```python
from build123d import *

# Parameters (mm, degrees)
F1_DEPTH  = 22
F0_R      = 28.575
F2_DEPTH  = 32
F3_W      = 22
F3_H      = 50
F4_DEPTH  = 114
F5_R      = 11.1
F6_DEPTH  = 32.001
F8_DEPTH  = 10
F9_DEPTH  = 64.001
F10_SIZE2 = 12
F10_SIZE  = 12


with BuildPart() as f1:
    # F0 (on Front) → F1 (new body, symmetric)
    with BuildSketch(Plane.XZ):
        with BuildLine():
            ThreePointArc((35.142567, 41), (49.05965, 22.564368), (54, 0))
            ThreePointArc((54, 0), (49.05965, -22.564368), (35.142567, -41))
            Line((35.142567, -41), (174, -41))
            Line((174, -41), (174, 41))
            Line((174, 41), (35.142567, 41))
        make_face()
    extrude(amount=F1_DEPTH, both=True)

    # F0 (on Front) → F2 (join, symmetric)
    with BuildSketch(Plane.XZ):
        with BuildLine():
            ThreePointArc((35.142567, -41), (49.05965, -22.564368), (54, 0))
            ThreePointArc((54, 0), (49.05965, 22.564368), (35.142567, 41))
            ThreePointArc((35.142567, 41), (-54, 0), (35.142567, -41))
        make_face()
        Circle(F0_R, mode=Mode.SUBTRACT)
        Circle(F0_R)
    extrude(amount=F2_DEPTH, both=True)

    # F3 (on face) → F4 (cut)
    with BuildSketch(Plane.YZ.offset(174)):
        with Locations((-11, 0)):
            Rectangle(F3_W, F3_H)
    extrude(amount=-F4_DEPTH, mode=Mode.SUBTRACT)

    # F5 (on face) → F6 (cut, through all)
    with BuildSketch(Plane.XZ):
        with Locations((139, 0)):
            Circle(F5_R)
        with Locations((89, 0)):
            Circle(F5_R)
    extrude(amount=-F6_DEPTH, mode=Mode.SUBTRACT)

    # F7 (on face) → F8 (join)
    with BuildSketch(Plane.XZ.offset(32)):
        with BuildLine():
            ThreePointArc((-23.675528, -16), (-28.575, 0), (-23.675528, 16))
            Line((-23.675528, 16), (-51.575188, 16))
            ThreePointArc((-51.575188, 16), (-54, 0), (-51.575188, -16))
            Line((-51.575188, -16), (-23.675528, -16))
        make_face()
        with BuildLine():
            ThreePointArc((23.675528, 16), (27.322691, 8.366672), (28.575, 0))
            ThreePointArc((28.575, 0), (27.322691, -8.366672), (23.675528, -16))
            Line((23.675528, -16), (51.575188, -16))
            ThreePointArc((51.575188, -16), (53.390356, -8.091349), (54, 0))
            ThreePointArc((54, 0), (53.390356, 8.091349), (51.575188, 16))
            Line((51.575188, 16), (23.675528, 16))
        make_face()
    extrude(amount=F8_DEPTH)

    # F7 (on face) → F9 (cut, through all)
    with BuildSketch(Plane.XZ.offset(32)):
        with BuildLine():
            ThreePointArc((23.675528, -16), (27.322691, -8.366672), (28.575, 0))
            ThreePointArc((28.575, 0), (27.322691, 8.366672), (23.675528, 16))
            ThreePointArc((23.675528, 16), (0, 28.575), (-23.675528, 16))
            ThreePointArc((-23.675528, 16), (-28.575, 0), (-23.675528, -16))
            ThreePointArc((-23.675528, -16), (0, -28.575), (23.675528, -16))
        make_face()
    extrude(amount=-F9_DEPTH, mode=Mode.SUBTRACT)

    # F10
    f10_edges = [f1.edges().sort_by_distance(p)[0] for p in [
        (174, -22, -33),
        (174, -22, 33),
    ]]
    chamfer(f10_edges, length=F10_SIZE, length2=F10_SIZE2)


solid = f1.part
```
Read the model definition and answer for the solid it produces. Units are mm, in the model's axes. A direction names the side the tool comes from. Coordinates: 2 decimals unless noted, no trailing zeros. Loops run counter-clockwise (first coordinate to the right, second up) from the corner with the lowest first, then second, coordinate; pieces in that order, holes last. Notation, with made-up numbers: (26.25, -12.5) - (43.25, -12.5) arc R15 ccw to (43.25, 13.5) - close; hole circle Ø3 at (72.25, 10.5). An arc over 180 degrees is marked (long way). Answer in a Markdown table with one row per item.
1. Given pin 1 (11 mm diameter, centred on x = 42, y = -35, fed in from -Z); pin 2 (19 mm diameter, centred on x = 11.5, z = 31.5, fed in from -Y); pin 3 (8 mm diameter, centred on x = -18, y = 23, fed in from -Z), each flat-ended and moving along its own axis, determine where each tip first touches the part or whether it passes through.
Conclusion:
| item | result |
|---|---|
| pin 1 | stops at z = -38.96 |
| pin 2 | stops at y = -32 |
| pin 3 | stops at z = -52.15 |
2. Straight lines are drawn through the part: line 1 (Z direction, x = 139, y = 8.75); line 2 (Y direction, x = 6, z = 31); line 3 (Z direction, x = 95, y = -14). For each, find the intervals that lie inside material, in ascending order.
Conclusion:
| item | result |
|---|---|
| line 1 | z = -41 to -11.1, 11.1 to 41 |
| line 2 | y = -32 to 32 |
| line 3 | z = -41 to -25, 25 to 41 |
3. Find section D-D, the plane y = 15. Write down the section's boundary in (x, z) (3 decimals), then the cut area to 3 significant figures.
Conclusion:
| item | result |
|---|---|
| outline | (35.143, -41) - (174, -41) - (174, 41) - (35.143, 41) arc R54 ccw (long way) to start; hole (23.676, -16) arc R28.575 ccw to (28.575, 0) arc R28.575 ccw to (23.676, 16) arc R28.575 ccw (long way) to start; hole circle Ø22.2 at (89, 0); hole circle Ø22.2 at (139, 0) |
| area | 16,100 mm² |
4. Determine the mould class of faces 5 (the face through (-1, -32, -35)), 6 (the face through (118, 0, 0)), 7 (the face through (127.91, 10.85, 0.49)), 8 (the face through (104, 0, -41)) for opening direction Z: +Z half, -Z half, draft (parallel to the pull), parting line (faces both ways), or undercut.
Conclusion:
| item | result |
|---|---|
| face 5 | draft |
| face 6 | undercut |
| face 7 | undercut |
| face 8 | -Z half |
5. Find section B-B, the plane y = -12.5. Write down the section's boundary in (x, z) (3 decimals), then the cut area to 3 significant figures.
Conclusion:
| item | result |
|---|---|
| outline | (35.143, -41) - (171.5, -41) - (171.5, -25) - (60, -25) - (60, 25) - (171.5, 25) - (171.5, 41) - (35.143, 41) arc R54 ccw (long way) to start; hole (23.676, -16) arc R28.575 ccw to (28.575, 0) arc R28.575 ccw to (23.676, 16) arc R28.575 ccw (long way) to start |
| area | 11,100 mm² |
6. Find section A-A, the plane x = 89. Write down the section's boundary in (y, z).
Conclusion:
| item | result |
|---|---|
| outline | (-22, -41) - (22, -41) - (22, -11.1) - (0, -11.1) - (0, -25) - (-22, -25) - close; (-22, 25) - (0, 25) - (0, 11.1) - (22, 11.1) - (22, 41) - (-22, 41) - close |
7. Which of the six approach directions +Z, -Z, +X, -X, +Y, -Y give full straight-line access (tool end or side, diameter ignored) to faces 1 (the face through (38, -37, 16)), 2 (the face through (106, 0, 41)), 3 (the face through (60, -11, 0)), 4 (the face through (-38, -37, -16))?
Conclusion:
| item | result |
|---|---|
| face 1 | +Z, +X, -X, -Y |
| face 2 | +Z, +X, +Y, -Y |
| face 3 | +X, -Y |
| face 4 | -Z, +X, -X, -Y |
8. Find section C-C, the plane z = -3. Write down the section's boundary in (x, y), then the cut area to 3 significant figures.
Conclusion:
| item | result |
|---|---|
| outline | (-53.92, -42) - (-28.42, -42) - (-28.42, 32) - (-53.92, 32) - close; (28.42, -42) - (53.92, -42) - (53.92, -22) - (60, -22) - (60, 0) - (78.31, 0) - (78.31, 22) - (53.92, 22) - (53.92, 32) - (28.42, 32) - close; (99.69, 0) - (128.31, 0) - (128.31, 22) - (99.69, 22) - close; (149.69, 0) - (174, 0) - (174, 22) - (149.69, 22) - close |
| area | 5,610 mm² |
